Answer from the drawing. Dimensions are ordinates in mm from the lowest x, y and z of the part. Round coordinates to 2 decimals unless told otherwise and drop trailing zeros. Write each loop counter-clockwise with the first axis right and the second up, starting at its lowest first coordinate (ties: lowest second). Pieces come first, ordered by that corner, then holes. Notation, with made-up numbers: (6.25, 69) - (35.25, 69) arc R28 cw to (35.25, 89) - close; hole circle Ø2 at (19.5, 52.5). An arc over 180 degrees is marked (long way). One line per item, written item: value. Start each with the question number.
(1) A cutting plane is placed at D-D, the plane x = 77.5. Determine the outline of the cut face in (y, z).
(2) Find the intervals of material crossed by L1, parallel to Z at x = 49, y = 11.5; L2, parallel to X at y = 6.5, z = 134.5; L3, parallel to Z at x = 58, y = 4, in increasing order.
(3) A cutting plane is placed at A-A, the plane z = 100. Determine the outline of the cut face in (x, y), plus the area to 3 significant figures.
(4) A cutting plane is placed at C-C, the plane y = 2.5. Determine the outline of the cut face in (x, z).
(5) A cutting plane is placed at B-B, the plane x = 100. Determine the outline of the cut face in (y, z).
(6) Flat-ended cylindrical pins translate along their axes: pin 1 Ø9.5 at (x, z) = (181.754, 100) entering from -Y; pin 2 Ø3 at (x, y) = (51, 7) entering from -Z; pin 3 Ø6.5 at (y, z) = (6.5, 106.5) entering from +X; pin 4 Ø6 at (x, y) = (31, 9.5) entering from +Z. Find the tip coordinate at first contact, or state that the pin passes through.
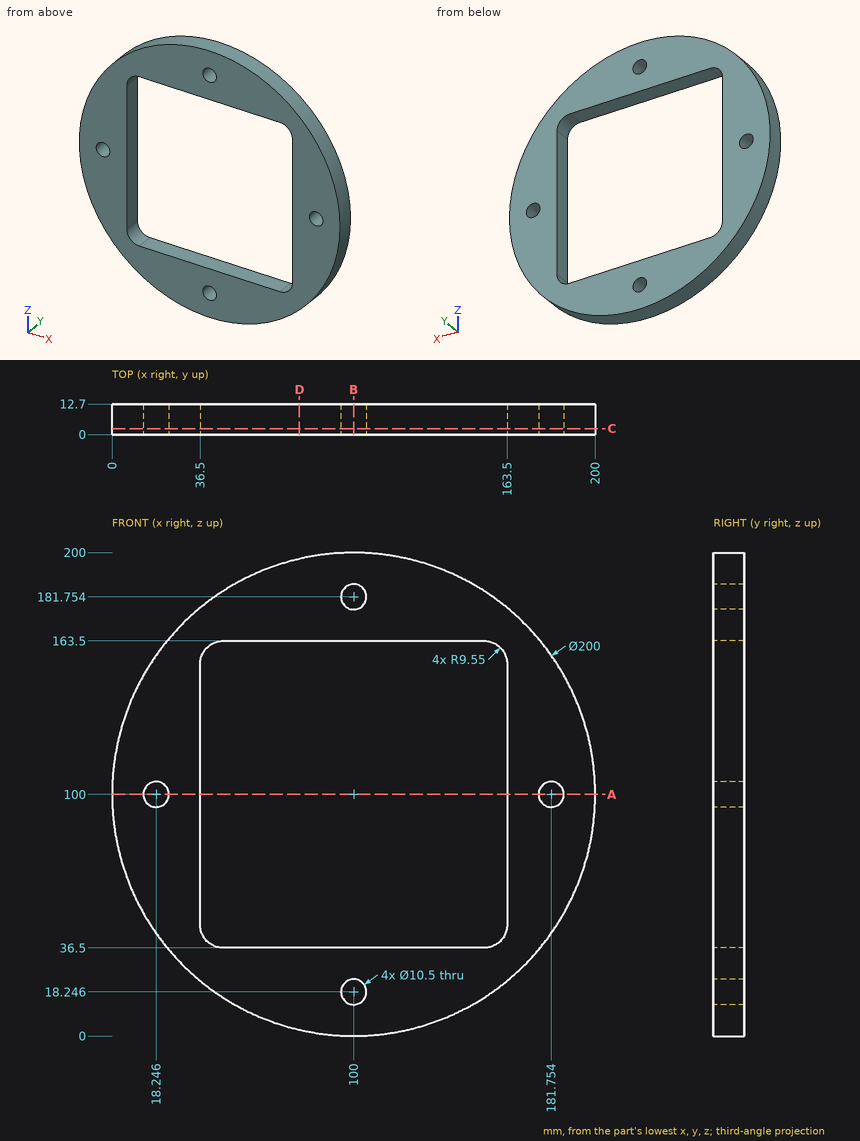
Here are the results:
1. outline: (0, 2.56) - (12.7, 2.56) - (12.7, 36.5) - (0, 36.5) - close; (0, 163.5) - (12.7, 163.5) - (12.7, 197.44) - (0, 197.44) - close
2. L1: 13.98 to 36.5, 163.5 to 186.02
2. L2: 6.14 to 36.5, 163.5 to 193.86
2. L3: 9.25 to 36.5, 163.5 to 190.75
3. outline: (0, 0) - (13, 0) - (13, 12.7) - (0, 12.7) - close; (23.5, 0) - (36.5, 0) - (36.5, 12.7) - (23.5, 12.7) - close; (163.5, 0) - (176.5, 0) - (176.5, 12.7) - (163.5, 12.7) - close; (187, 0) - (200, 0) - (200, 12.7) - (187, 12.7) - close
3. area: 660 mm²
4. outline: circle Ø200 at (100, 100); hole circle Ø10.5 at (18.25, 100); hole (36.5, 46.05) arc R9.55 ccw to (46.05, 36.5) - (153.95, 36.5) arc R9.55 ccw to (163.5, 46.05) - (163.5, 153.95) arc R9.55 ccw to (153.95, 163.5) - (46.05, 163.5) arc R9.55 ccw to (36.5, 153.95) - close; hole circle Ø10.5 at (100, 18.25); hole circle Ø10.5 at (100, 181.75); hole circle Ø10.5 at (181.75, 100)
5. outline: (0, 0) - (12.7, 0) - (12.7, 13) - (0, 13) - close; (0, 23.5) - (12.7, 23.5) - (12.7, 36.5) - (0, 36.5) - close; (0, 163.5) - (12.7, 163.5) - (12.7, 176.5) - (0, 176.5) - close; (0, 187) - (12.7, 187) - (12.7, 200) - (0, 200) - close
6. pin 1: through
6. pin 2: z = 12
6. pin 3: x = 199.95
6. pin 4: z = 175.13
